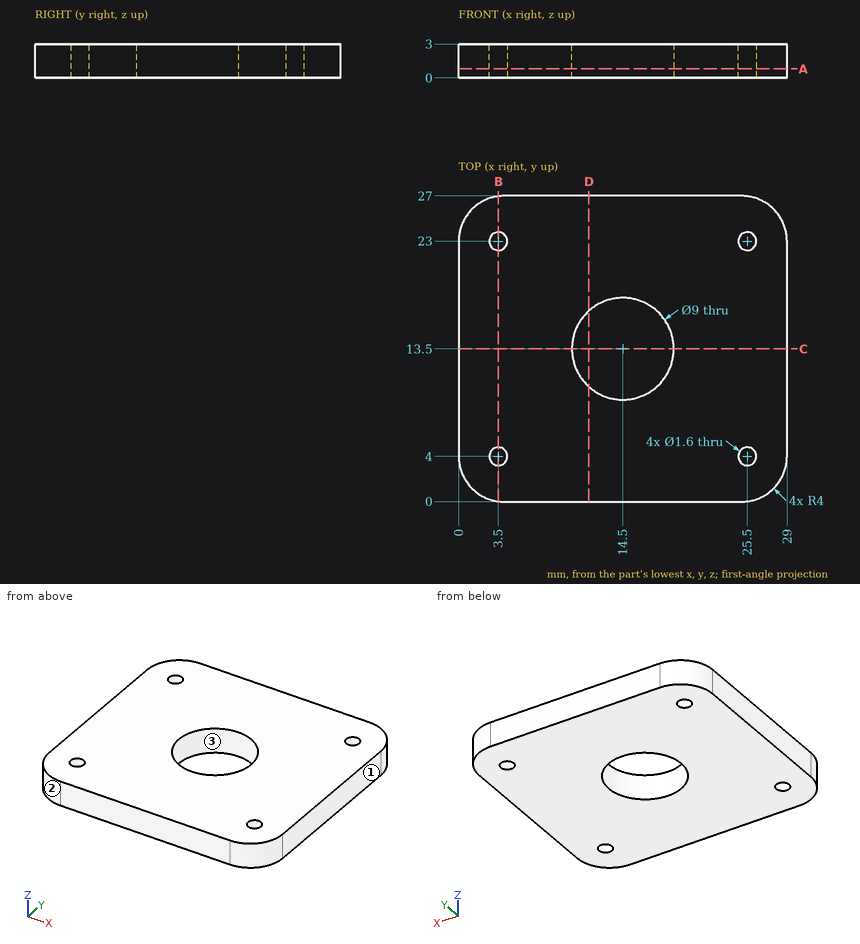
Geometry: see drawing. Coordinates: mm, zero at the bounding-box minimum. Give positions to 0.01 mm unless a question says otherwise; leave off trailing zeros. Loops run counter-clockwise (first coordinate to the right, second up) from the corner with the lowest first, then second, coordinate; pieces in that order, holes last. Notation, with made-up numbers: (54, 39.25) - (82, 39.25) arc R12 ccw to (82, 50.25) - close; hole circle Ø8 at (82, 79.25). An arc over 180 degrees is marked (long way). Use CSV: the item, a comma, the result in double quotes.
1) Pin query (flat end, axial travel): P1, Ø2.5, axis at x = 3.5, y = 4, coming from the +Z side. Return the tip coordinate at first contact, or that it passes through.
Worked out:
P1,"stops at z = 3"
2) Cut plane C-C (y = 13.5). Output: boundary loops of the cut face in (x, z), and give its area (3 significant figures).
Worked out:
outline,"(0, 0) - (10, 0) - (10, 3) - (0, 3) - close; (19, 0) - (29, 0) - (29, 3) - (19, 3) - close"
area,"60.0 mm^2"
3) Cut plane A-A (z = 0.8). Output: boundary loops of the cut face in (x, y).
Worked out:
outline,"(0, 4) arc R4 ccw to (4, 0) - (25, 0) arc R4 ccw to (29, 4) - (29, 23) arc R4 ccw to (25, 27) - (4, 27) arc R4 ccw to (0, 23) - close; hole circle Ø1.6 at (3.5, 4); hole circle Ø1.6 at (3.5, 23); hole circle Ø9 at (14.5, 13.5); hole circle Ø1.6 at (25.5, 4); hole circle Ø1.6 at (25.5, 23)"
4) Line query: line 1 (Y direction, x = 3.5, z = 2.1); line 2 (Y direction, x = 14.5, z = 0.9); line 3 (Y direction, x = 18, z = 0.5). Output: solid intervals per line, ascending.
Worked out:
line 1,"y = 0.03 to 3.2, 4.8 to 22.2, 23.8 to 26.97"
line 2,"y = 0 to 9, 18 to 27"
line 3,"y = 0 to 10.67, 16.33 to 27"
5) Mould query, pull axis Y, two halves, no side actions, for the marked faces 1, 2 and 3. Classes: +Y half, -Y half, draft (parallel to the pull), parting line (faces both ways), or undercut.
Worked out:
face 1,"draft"
face 2,"-Y half"
face 3,"undercut"
6) Cut plane D-D (x = 11.5). Output: boundary loops of the cut face in (y, z).
Worked out:
outline,"(0, 0) - (10.15, 0) - (10.15, 3) - (0, 3) - close; (16.85, 0) - (27, 0) - (27, 3) - (16.85, 3) - close"
7) Cut plane B-B (x = 3.5). Output: boundary loops of the cut face in (y, z), and give its area (3 significant figures).
Worked out:
outline,"(0.03, 0) - (3.2, 0) - (3.2, 3) - (0.03, 3) - close; (4.8, 0) - (22.2, 0) - (22.2, 3) - (4.8, 3) - close; (23.8, 0) - (26.97, 0) - (26.97, 3) - (23.8, 3) - close"
area,"71.2 mm^2"
